Geometry: final body of the model. Coordinates: model frame, mm. Round coordinates to 2 decimals unless told otherwise and drop trailing zeros. Loops run counter-clockwise (first coordinate to the right, second up) from the corner with the lowest first, then second, coordinate; pieces in that order, holes last. Notation, with made-up numbers: M 75.5,59 L 114.5,59 A20 cw 114.5,90 Z; hole C -3,43 d6. An arc over 180 degrees is marked long. Return JSON: item names as keys, results as strings.
from build123d import *

# Parameters (mm, degrees)
F1_DEPTH = 9.525


with BuildPart() as f1:
    # F0 (on Front) → F1 (new body)
    with BuildSketch(Plane.XZ):
        Polygon((46.425866, 118.218941), (0, 42.89867), (-46.425841, 118.218941), (-9.642704, 118.218941), (-9.642704, 262.373212), (-275.353094, 262.373212), (-275.353094, 118.218941), (-238.419894, 118.218941), (-379.852555, -117.502153), (-436.247438, -117.502153), (-436.247438, -262.373186), (-166.750771, -262.373186), (-166.750771, -117.675508), (-208.63687, -117.675508), (-141.304645, -6.354039), (-122.033462, -38.525171), (-147.4629, -38.525171), (-147.4629, -182.446219), (147.4629, -182.446219), (147.4629, -38.525171), (122.033487, -38.525171), (141.30467, -6.354039), (208.636895, -117.675508), (166.750797, -117.675508), (166.750797, -262.373186), (436.247438, -262.373186), (436.247438, -117.502153), (379.852555, -117.502153), (238.419919, 118.218941), (275.35312, 118.218941), (275.35312, 262.373212), (9.642729, 262.373212), (9.642729, 118.218941), align=None)
    extrude(amount=F1_DEPTH)


solid = f1.part
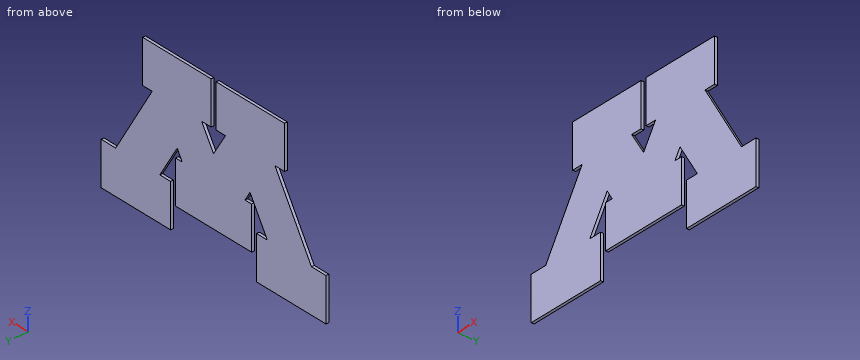
Q1. Material intervals for L1, parallel to X at y = -2.5, z = -169.5; L2, parallel to X at y = -9, z = -195; L3, parallel to X at y = -1.75, z = -58, sorted ascending.
Determined:
{"L1": "x = -436.25 to -166.75, -147.46 to 147.46, 166.75 to 436.25", "L2": "x = -436.25 to -166.75, 166.75 to 436.25", "L3": "x = -344.15 to -172.54, -147.46 to 147.46, 172.54 to 344.15"}
Q2. Pin query (flat end, axial travel): pin 1 (5 mm diameter, centred on y = -4, z = 220.5, fed in from +X); pin 2 (3 mm diameter, centred on y = -6.5, z = 208, fed in from -X); pin 3 (3 mm diameter, centred on x = -401.5, y = -4.5, fed in from +Z); pin 4 (10 mm diameter, centred on x = -22.5, z = 108.5, fed in from +Y). Return the tip coordinate at first contact, or that it passes through.
Determined:
{"pin 1": "stops at x = 275.35", "pin 2": "stops at x = -275.35", "pin 3": "stops at z = -117.5", "pin 4": "passes through"}
Q3. Section query B-B (x = -29). Output: boundary loops of the cut face in (y, z) (3 decimals), plus the area to 3 significant figures.
Determined:
{"outline": "M -9.525,-182.446 L 0,-182.446 L 0,89.948 L -9.525,89.948 Z; M -9.525,118.219 L 0,118.219 L 0,262.373 L -9.525,262.373 Z", "area": "3,970 mm^2"}
Q4. Section query C-C (z = -67.5). Output: boundary loops of the cut face in (x, y) (1 decimal), plus the area to 3 significant figures.
Determined:
{"outline": "M -349.9,-9.5 L -178.3,-9.5 L -178.3,0 L -349.9,0 Z; M -147.5,-9.5 L 147.5,-9.5 L 147.5,0 L -147.5,0 Z; M 178.3,-9.5 L 349.9,-9.5 L 349.9,0 L 178.3,0 Z", "area": "6,080 mm^2"}
Q5. Section query A-A (z = 230.5). Output: boundary loops of the cut face in (x, y) (3 decimals).
Determined:
{"outline": "M -275.353,-9.525 L -9.643,-9.525 L -9.643,0 L -275.353,0 Z; M 9.643,-9.525 L 275.353,-9.525 L 275.353,0 L 9.643,0 Z"}
